Here's how the part is built. I have some questions about the finished solid (model axes, mm). Round coordinates to 2 decimals unless told otherwise and drop trailing zeros. Loops run counter-clockwise (first coordinate to the right, second up) from the corner with the lowest first, then second, coordinate; pieces in that order, holes last. Notation, with made-up numbers: (-23, 69.25) -> (33, 69.25) arc R20 cw to (33, 98.25) -> close; hole circle Ø5 at (78, 1.5). An arc over 180 degrees is marked (long way). One line per item, written item: value. Start each with the question number.
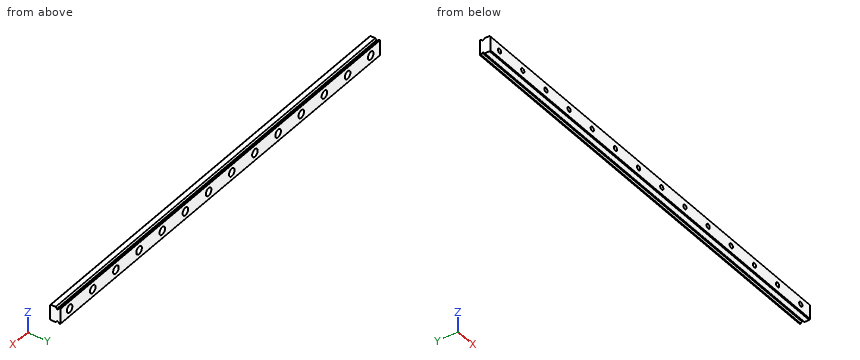
```python
from build123d import *

# Parameters (mm, degrees)
SKETCH_1_W                   = 345
SKETCH_1_H                   = 12
EXTRUDE_1_DEPTH              = 8
CUT_EXTRUDE_1_DEPTH          = 346.07535409
CUT_EXTRUDE_2_DEPTH          = 346.07535409
CUT_EXTRUDE_3_DEPTH          = 346.07535409
CUT_EXTRUDE_4_DEPTH          = 346.07535409
CUT_EXTRUDE_5_DEPTH          = 346.07535409
CUT_EXTRUDE_6_DEPTH          = 346.07535409
HOLE_WIZARD_M3_1_D           = 3.5
HOLE_WIZARD_M3_1_CBORE_D     = 5.9999
HOLE_WIZARD_M3_1_CBORE_DEPTH = 4.5
CHAMFER_1_SIZE               = 0.6
FILLET_1_R                   = 0.2


with BuildPart() as part:
    # 草图1 → 凸台-拉伸1 (new body)
    with BuildSketch(Plane(origin=(0, 4, 0), x_dir=(1, 0, 0), z_dir=(0, 1, 0))):
        Rectangle(SKETCH_1_W, SKETCH_1_H)
    extrude(amount=-EXTRUDE_1_DEPTH)

    # 草图2 → 切除-拉伸1 (cut, through all)
    with BuildSketch(Plane(origin=(172.5, 0, 0), x_dir=(0, 0, -1), z_dir=(1, 0, 0))):
        with BuildLine():
            Line((6, 1.51), (6, 2.01))
            Line((6, 2.01), (4.8, 2.01))
            ThreePointArc((4.8, 2.01), (4.55, 1.76), (4.8, 1.51))
            Line((4.8, 1.51), (6, 1.51))
        make_face()
    extrude(amount=-CUT_EXTRUDE_1_DEPTH, mode=Mode.SUBTRACT)

    # 草图3 → 切除-拉伸2 (cut, through all)
    with BuildSketch(Plane(origin=(172.5, 0, 0), x_dir=(0, 0, -1), z_dir=(1, 0, 0))):
        with BuildLine():
            Line((6, 2.01), (6, 3.111111))
            ThreePointArc((6, 3.111111), (5.367595703, 2.693428684), (5.04, 2.01))
            Line((5.04, 2.01), (6, 2.01))
        make_face()
    extrude(amount=-CUT_EXTRUDE_2_DEPTH, mode=Mode.SUBTRACT)

    # 草图4 → 切除-拉伸3 (cut, through all)
    with BuildSketch(Plane(origin=(172.5, 0, 0), x_dir=(0, 0, -1), z_dir=(1, 0, 0))):
        with BuildLine():
            Line((6, 1.51), (5.04, 1.51))
            ThreePointArc((5.04, 1.51), (5.367595703, 0.826571316), (6, 0.408889))
            Line((6, 0.408889), (6, 1.51))
        make_face()
    extrude(amount=-CUT_EXTRUDE_3_DEPTH, mode=Mode.SUBTRACT)

    # 草图5 → 切除-拉伸4 (cut, through all)
    with BuildSketch(Plane(origin=(172.5, 0, 0), x_dir=(0, 0, -1), z_dir=(1, 0, 0))):
        with BuildLine():
            Line((-6, 2.01), (-6, 1.51))
            Line((-6, 1.51), (-4.8, 1.51))
            ThreePointArc((-4.8, 1.51), (-4.55, 1.76), (-4.8, 2.01))
            Line((-4.8, 2.01), (-6, 2.01))
        make_face()
    extrude(amount=-CUT_EXTRUDE_4_DEPTH, mode=Mode.SUBTRACT)

    # 草图6 → 切除-拉伸5 (cut, through all)
    with BuildSketch(Plane(origin=(172.5, 0, 0), x_dir=(0, 0, -1), z_dir=(1, 0, 0))):
        with BuildLine():
            Line((-6, 1.51), (-6, 0.408889))
            ThreePointArc((-6, 0.408889), (-5.367595703, 0.826571316), (-5.04, 1.51))
            Line((-5.04, 1.51), (-6, 1.51))
        make_face()
    extrude(amount=-CUT_EXTRUDE_5_DEPTH, mode=Mode.SUBTRACT)

    # 草图7 → 切除-拉伸6 (cut, through all)
    with BuildSketch(Plane(origin=(172.5, 0, 0), x_dir=(0, 0, -1), z_dir=(1, 0, 0))):
        with BuildLine():
            Line((-6, 2.01), (-5.04, 2.01))
            ThreePointArc((-5.04, 2.01), (-5.367595703, 2.693428684), (-6, 3.111111))
            Line((-6, 3.111111), (-6, 2.01))
        make_face()
    extrude(amount=-CUT_EXTRUDE_6_DEPTH, mode=Mode.SUBTRACT)

    # M3 六角头机械螺钉的柱形沉头孔1 (through all)
    with Locations(Plane(origin=(0, 4, 0), x_dir=(1, 0, 0), z_dir=(0, 1, 0))):
        with Locations((-162.5, 0), (-137.5, 0), (-112.5, 0), (-87.5, 0), (-62.5, 0), (-37.5, 0), (-12.5, 0), (12.5, 0), (37.5, 0), (62.5, 0), (87.5, 0), (112.5, 0), (137.5, 0), (162.5, 0)):
            CounterBoreHole(HOLE_WIZARD_M3_1_D / 2, HOLE_WIZARD_M3_1_CBORE_D / 2, HOLE_WIZARD_M3_1_CBORE_DEPTH)

    # 倒角1
    chamfer_1_edges = [part.edges().sort_by_distance(p)[0] for p in [
        (0, -4, -6),
        (0, -4, 6),
    ]]
    chamfer(chamfer_1_edges, length=CHAMFER_1_SIZE)

    # 圆角1
    fillet_1_edges = [part.edges().sort_by_distance(p)[0] for p in [
        (0, 2.01, -5.04),
        (0, 3.111111, -6),
        (0, 0.408889, -6),
        (0, 1.51, -5.04),
        (0, 4, -6),
        (0, 4, 6),
        (0, 1.51, 5.04),
        (0, 0.408889, 6),
        (0, 3.111111, 6),
        (0, 2.01, 5.04),
    ]]
    fillet(fillet_1_edges, radius=FILLET_1_R)


solid = part.part
```
Q1. If I drill on line 1 along Z through (x, y) = (-137.5, 3); line 2 along Y through (x, z) = (-142.5, -4.75); line 3 along Z through (x, y) = (112.5, -1.5), over which ranges is the centre line in solid material (lowest first)?
Q2. I want a section at A-A on x = -70.5. Please give me the cut outline in (y, z), plus the area to 3 significant figures.
Q3. Will this pin go through, and if not, where does the flat tip stop? P1, Ø1.8, axis at x = 111.5, z = -0.5, coming from the +Y side.
Answers below:
1. line 1: z = -5.75 to -3, 3 to 5.75
1. line 2: y = -4 to 1.52, 2 to 4
1. line 3: z = -6 to -1.75, 1.75 to 6
2. outline: (-4, -5.4) -> (-3.4, -6) -> (0.27, -6) arc R0.2 ccw to (0.45, -5.88) arc R1.42 cw to (1.37, -5.07) arc R0.2 ccw to (1.51, -4.88) -> (1.51, -4.8) arc R0.25 cw to (2.01, -4.8) -> (2.01, -4.88) arc R0.2 ccw to (2.15, -5.07) arc R1.42 cw to (3.07, -5.88) arc R0.2 ccw to (3.25, -6) -> (3.8, -6) arc R0.2 ccw to (4, -5.8) -> (4, 5.8) arc R0.2 ccw to (3.8, 6) -> (3.25, 6) arc R0.2 ccw to (3.07, 5.88) arc R1.42 cw to (2.15, 5.07) arc R0.2 ccw to (2.01, 4.88) -> (2.01, 4.8) arc R0.25 cw to (1.51, 4.8) -> (1.51, 4.88) arc R0.2 ccw to (1.37, 5.07) arc R1.42 cw to (0.45, 5.88) arc R0.2 ccw to (0.27, 6) -> (-3.4, 6) -> (-4, 5.4) -> close
2. area: 91.3 mm^2
3. P1: stops at y = -0.5
